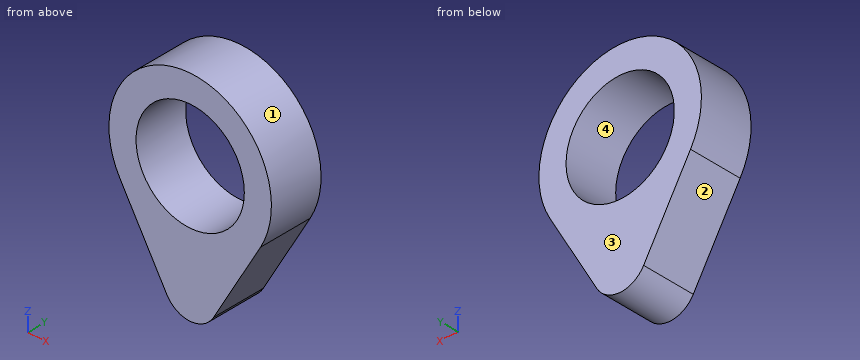
from build123d import *

# Parameters (mm, degrees)
F1_R     = 12.7
F2_DEPTH = 12.7


with BuildPart() as f2:
    # F1 (on offset) → F2 (new body)
    with BuildSketch(Plane.XZ.offset(63.5)):
        with BuildLine():
            Line((5.499261, -28.575), (16.497784, -9.525))
            ThreePointArc((16.497784, -9.525), (0, 19.05), (-16.497784, -9.525))
            Line((-16.497784, -9.525), (-5.499261, -28.575))
            ThreePointArc((-5.499261, -28.575), (0, -31.75), (5.499261, -28.575))
        make_face()
        Circle(F1_R, mode=Mode.SUBTRACT)
    extrude(amount=-F2_DEPTH)


solid = f2.part
Verification items for the finished model (mm, model axes). Face numbers are marked on the shaded views. Give positions to 0.01 mm unless a question says otherwise; leave off trailing zeros. Write each loop counter-clockwise with the first axis right and the second up, starting at its lowest first coordinate (ties: lowest second). Pieces come first, ordered by that corner, then holes. Notation, with made-up numbers: (22.5, -10) -> (68.5, -10) arc R20 cw to (68.5, -1) -> close; hole circle Ø10 at (-6, 34). An arc over 180 degrees is marked (long way). Use CSV: the item, a comma, the result in double quotes.
(1) Sectioned sample at C-C (y = -54.25). Record the cut outline in (x, z) (3 decimals), plus the area to 3 significant figures.
Derived:
outline,"(-16.498, -9.525) -> (-5.499, -28.575) arc R6.35 ccw to (5.499, -28.575) -> (16.498, -9.525) arc R19.05 ccw (long way) to start; hole circle Ø25.4 at (0, 0)"
area,"854 mm^2"
(2) Sectioned sample at D-D (z = -18). Record the cut outline in (x, y), plus the area to 3 significant figures.
Derived:
outline,"(-11.6, -63.5) -> (11.6, -63.5) -> (11.6, -50.8) -> (-11.6, -50.8) -> close"
area,"295 mm^2"
(3) Go/stop test with flat-tipped pins: pin 1 (4 mm diameter, centred on y = -56, z = -13, fed in from +X); pin 2 (5 mm diameter, centred on x = -11, z = -2, fed in from -Y); pin 3 (4 mm diameter, centred on y = -60.5, z = -22.5, fed in from -X); pin 4 (1.5 mm diameter, centred on x = 8, y = -59, fed in from +Z). Record where each tip stops, or that it passes through.
Derived:
pin 1,"stops at x = 15.65"
pin 2,"stops at y = -63.5"
pin 3,"stops at x = -10.16"
pin 4,"stops at z = 17.62"
(4) Sectioned sample at B-B (x = 0). Record the cut outline in (y, z), plus the area to 3 significant figures.
Derived:
outline,"(-63.5, -31.75) -> (-50.8, -31.75) -> (-50.8, -12.7) -> (-63.5, -12.7) -> close; (-63.5, 12.7) -> (-50.8, 12.7) -> (-50.8, 19.05) -> (-63.5, 19.05) -> close"
area,"323 mm^2"
(5) Material ranges on L1, parallel to X at y = -53.75, z = 0.5; L2, parallel to X at y = -60, z = -2; L3, parallel to Z at x = 4, y = -59, recorded low to high.
Derived:
L1,"x = -19.04 to -12.69, 12.69 to 19.04"
L2,"x = -18.94 to -12.54, 12.54 to 18.94"
L3,"z = -30.33 to -12.05, 12.05 to 18.63"
(6) Release check for a two-part mould opening along Z. For the marked faces 1, 2, 3 and 4 record: +Z half, -Z half, draft (parallel to the pull), parting line (faces both ways), or undercut.
Derived:
face 1,"parting line"
face 2,"-Z half"
face 3,"draft"
face 4,"undercut"
(7) Sectioned sample at A-A (z = 0). Record the cut outline in (x, y).
Derived:
outline,"(-19.05, -63.5) -> (-12.7, -63.5) -> (-12.7, -50.8) -> (-19.05, -50.8) -> close; (12.7, -63.5) -> (19.05, -63.5) -> (19.05, -50.8) -> (12.7, -50.8) -> close"
